Drawing for the job (mm, zero at the part's lowest x, y, z). A direction names the side the tool comes from. Coordinates: 2 decimals unless noted, no trailing zeros. Loops run counter-clockwise (first coordinate to the right, second up) from the corner with the lowest first, then second, coordinate; pieces in that order, holes last. Notation, with made-up numbers: (-22.75, 36.5) - (-0.75, 36.5) arc R23 cw to (-0.75, 64.5) - close; hole circle Ø8 at (-29, -39). An arc over 180 degrees is marked (long way). Put each result on its own line as item: value.
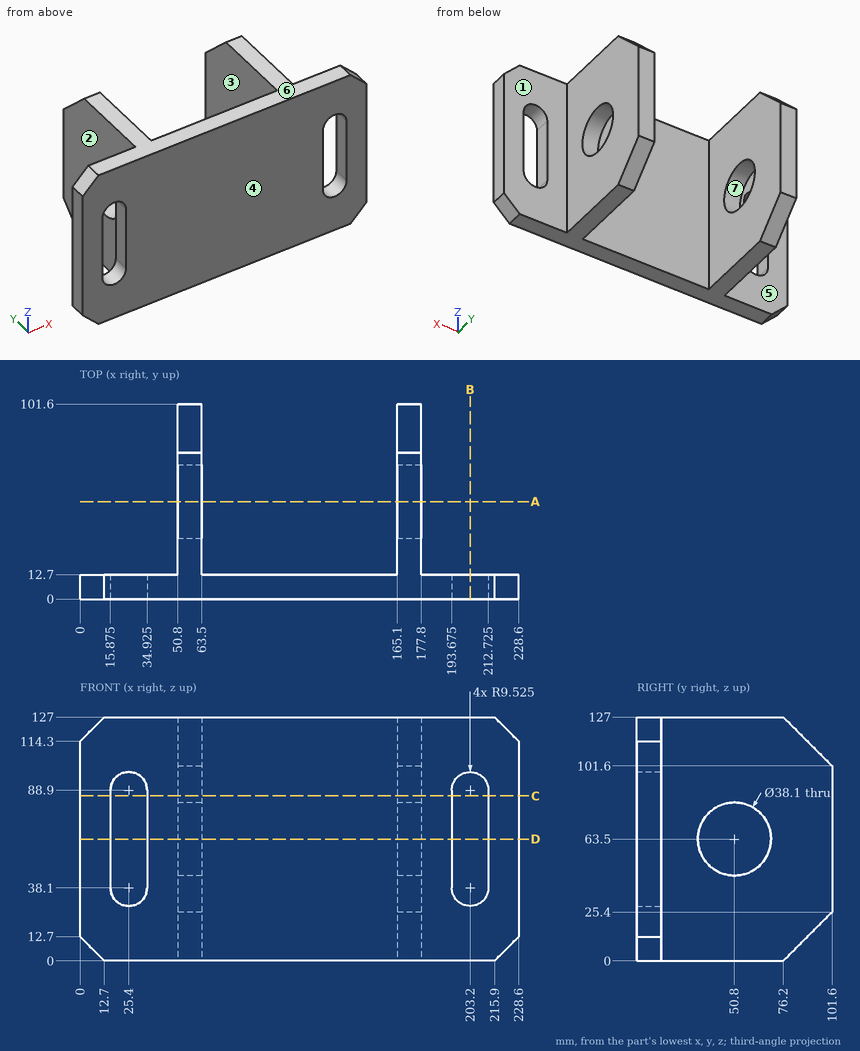
Q1. Tool access for the marked faces 1, 2, 3 and 4: list every direction of +Z, -Z, +X, -X, +Y, -Y with a clear straight run to the whole face (end or side of a thin tool).
Determined:
face 1: +Z, -Z, +X, +Y
face 2: +Z, -Z, -X, +Y
face 3: +Z, -Z, +Y
face 4: +Z, -Z, +X, -X, -Y
Q2. Slice it at A-A, the plane y = 50.8. Give the cut face in (x, z), then the cut area to 3 significant figures.
Determined:
outline: (50.8, 0) - (63.5, 0) - (63.5, 44.45) - (50.8, 44.45) - close; (50.8, 82.55) - (63.5, 82.55) - (63.5, 127) - (50.8, 127) - close; (165.1, 0) - (177.8, 0) - (177.8, 44.45) - (165.1, 44.45) - close; (165.1, 82.55) - (177.8, 82.55) - (177.8, 127) - (165.1, 127) - close
area: 2,260 mm2
Q3. Slice it at B-B, the plane x = 203.2. Give the cut face in (y, z) (3 decimals), then the cut area to 3 significant figures.
Determined:
outline: (0, 0) - (12.7, 0) - (12.7, 28.575) - (0, 28.575) - close; (0, 98.425) - (12.7, 98.425) - (12.7, 127) - (0, 127) - close
area: 726 mm2
Q4. Slice it at C-C, the plane z = 86. Give the cut face in (x, y) (3 decimals).
Determined:
outline: (0, 0) - (15.875, 0) - (15.875, 12.7) - (0, 12.7) - close; (34.925, 0) - (193.675, 0) - (193.675, 12.7) - (177.8, 12.7) - (177.8, 101.6) - (165.1, 101.6) - (165.1, 12.7) - (63.5, 12.7) - (63.5, 101.6) - (50.8, 101.6) - (50.8, 12.7) - (34.925, 12.7) - close; (212.725, 0) - (228.6, 0) - (228.6, 12.7) - (212.725, 12.7) - close
Q5. Mould opens along Z. For the marked faces 5, 6 and 7 say: +Z half, -Z half, draft (parallel to the pull), parting line (faces both ways), or undercut.
Determined:
face 5: draft
face 6: +Z half
face 7: undercut
Q6. Wall check: L1, parallel to X at y = 72, z = 76; L2, parallel to Z at x = 173, y = 50; L3, parallel to Y at x = 174.5, z = 63.5. Give the ranges that are in metal, low to high. Write a range as from..to.
Determined:
L1: 50.8..63.5, 165.1..177.8
L2: 0..44.47, 82.53..127
L3: 0..31.75, 69.85..101.6
Q7. Slice it at D-D, the plane z = 63.5. Give the cut face in (x, y) (3 decimals).
Determined:
outline: (0, 0) - (15.875, 0) - (15.875, 12.7) - (0, 12.7) - close; (34.925, 0) - (193.675, 0) - (193.675, 12.7) - (177.8, 12.7) - (177.8, 31.75) - (165.1, 31.75) - (165.1, 12.7) - (63.5, 12.7) - (63.5, 31.75) - (50.8, 31.75) - (50.8, 12.7) - (34.925, 12.7) - close; (50.8, 69.85) - (63.5, 69.85) - (63.5, 101.6) - (50.8, 101.6) - close; (165.1, 69.85) - (177.8, 69.85) - (177.8, 101.6) - (165.1, 101.6) - close; (212.725, 0) - (228.6, 0) - (228.6, 12.7) - (212.725, 12.7) - close
Q8. Pin check, flat tips, straight feed: pin 1 Ø1.5 at (y, z) = (29, 37) entering from -X; pin 2 Ø5 at (x, z) = (103, 109.5) entering from +Y. Stop position of each tip, or through.
Determined:
pin 1: x = 50.8
pin 2: y = 12.7
